Verification items for the finished model (mm, model axes). Round coordinates to 2 decimals unless told otherwise and drop trailing zeros. Order: outer loops, then holes, each group sorted by start corner. A loop starts at its lowest first (then second) coordinate and runs counter-clockwise, first axis right, second up. Notation, with made-up numbers: (47, 73.5) -> (64, 73.5) arc R7 cw to (64, 81.5) -> close; hole circle Ø9 at (48.5, 27.5). An arc over 180 degrees is marked (long way). Put each result on its own line as item: value.
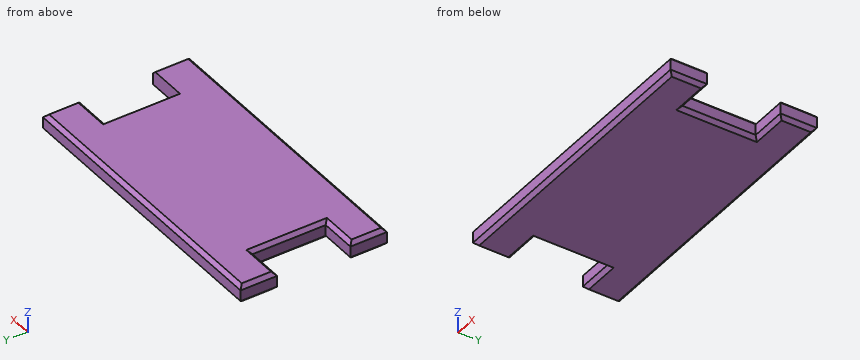
```python
from build123d import *

# Parameters (mm, degrees)
F1_DEPTH = 25
F2_SIZE  = 5
F3_SIZE  = 5
F5_SIZE  = 5


# Not quite as in the source:
# - a feature of the source that left no trace in its solid (it failed there, or was rolled back) is left out


with BuildPart() as f1:
    # F0 (on Top) → F1 (new body)
    with BuildSketch(Plane.XY):
        Polygon((0, 50), (0, 0), (400, 0), (400, 50), (350, 50), (350, 150), (400, 150), (400, 200), (0, 200), (0, 150), (50, 150), (50, 50), align=None)
    extrude(amount=F1_DEPTH)

    # F2
    f2_edges = [f1.edges().sort_by_distance(p)[0] for p in [
        (200, 0, 25),
    ]]
    chamfer(f2_edges, length=F2_SIZE)

    # F3
    f3_edges = [f1.edges().sort_by_distance(p)[0] for p in [
        (200, 200, 25),
    ]]
    chamfer(f3_edges, length=F3_SIZE)

    # F5
    f5_edges = [f1.edges().sort_by_distance(p)[0] for p in [
        (200, 0, 0),
        (200, 200, 0),
        (350, 100, 0),
        (375, 50, 0),
        (400, 25, 0),
        (400, 175, 0),
        (375, 150, 0),
        (0, 175, 0),
        (25, 150, 0),
        (50, 100, 0),
        (25, 50, 0),
        (0, 25, 0),
        (0, 172.5, 25),
        (25, 150, 25),
        (400, 172.5, 25),
        (50, 100, 25),
        (375, 150, 25),
        (25, 50, 25),
        (350, 100, 25),
        (0, 27.5, 25),
        (400, 27.5, 25),
    ]]
    chamfer(f5_edges, length=F5_SIZE)


solid = f1.part
```
Item 1: Sectioned sample at B-B, the plane z = 14.5. Record the boundary of the cut face in (x, y), then the cut area to 3 significant figures.
Geometry check:
outline: (0, 0) -> (400, 0) -> (400, 50) -> (350, 50) -> (350, 150) -> (400, 150) -> (400, 200) -> (0, 200) -> (0, 150) -> (50, 150) -> (50, 50) -> (0, 50) -> close
area: 70,000 mm2
Item 2: Depth check by flat-ended pin: pin 1 Ø12 at (y, z) = (93, 16) entering from -X; pin 2 Ø1 at (y, z) = (55.5, 6.5) entering from +X. Enter the tip coordinate at first touch or a pass-through.
Geometry check:
pin 1: x = 50
pin 2: x = 350
Item 3: Sectioned sample at A-A, the plane y = 118. Record the boundary of the cut face in (x, z), then the cut area to 3 significant figures.
Geometry check:
outline: (50, 5) -> (55, 0) -> (345, 0) -> (350, 5) -> (350, 20) -> (345, 25) -> (55, 25) -> (50, 20) -> close
area: 7,450 mm2
Item 4: Material ranges on line 1 along X through (y, z) = (51, 5); line 2 along X through (y, z) = (154, 3.25); line 3 along Z through (x, y) = (53, 53), recorded low to high.
Geometry check:
line 1: 50 to 350
line 2: 1.75 to 398.25
line 3: 2 to 23
